```python
from build123d import *

# Parameters (mm, degrees)
BOSS_EXTRUDE1_DEPTH = 10
SKETCH3_R           = 1.75
CUT_EXTRUDE1_DEPTH  = 12.874342087
FILLET2_R           = 1


with BuildPart() as part:
    # Sketch1 → Boss-Extrude1 (new body)
    with BuildSketch(Plane.XY):
        Polygon((-2.5, 0), (2.5, 0), (5, 3), (5, 4), (-5, 4), (-5, 3), align=None)
    extrude(amount=BOSS_EXTRUDE1_DEPTH)

    # Sketch3 → Cut-Extrude1 (cut, through all)
    with BuildSketch(Plane(origin=(0, 4, 0), x_dir=(1, 0, 0), z_dir=(0, 1, 0))):
        with Locations(Location((0, -5, 0), (0, 0, 270))):
            Circle(SKETCH3_R)
    extrude(amount=-CUT_EXTRUDE1_DEPTH, mode=Mode.SUBTRACT)

    # Fillet2
    # the kernel refuses this fillet: 1 mm, written as the material it takes off along each edge
    with BuildSketch(Plane(origin=(-5, 0, 10), x_dir=(0, 0, -1), z_dir=(1, 0, 0))) as fillet2_piece_1:
        with BuildLine():
            CenterArc((FILLET2_R, FILLET2_R), FILLET2_R, 180, 90)
            Line((0, FILLET2_R), (0, 0))
            Line((0, 0), (FILLET2_R, 0))
        make_face()
    extrude(amount=10, mode=Mode.SUBTRACT)
    with BuildSketch(Plane(origin=(0.899539001, -1.920553199, 10), x_dir=(-0.768221279597376, 0.6401843996644797, 0), z_dir=(0.6401843996644797, 0.768221279597376, 0))) as fillet2_piece_2:
        with BuildLine():
            CenterArc((FILLET2_R, -FILLET2_R), FILLET2_R, 90, 90)
            Line((0, -FILLET2_R), (0, 0))
            Line((0, 0), (FILLET2_R, 0))
        make_face()
    extrude(amount=8.905124838, mode=Mode.SUBTRACT)
    with BuildSketch(Plane(origin=(-6.600460999, 4.920553199, 10), x_dir=(0, 0, -1), z_dir=(0.6401843996644797, -0.768221279597376, 0))) as fillet2_piece_3:
        with BuildLine():
            CenterArc((FILLET2_R, FILLET2_R), FILLET2_R, 180, 90)
            Line((0, FILLET2_R), (0, 0))
            Line((0, 0), (FILLET2_R, 0))
        make_face()
    extrude(amount=8.905124838, mode=Mode.SUBTRACT)
    with BuildSketch(Plane(origin=(7.5, 4, 10), x_dir=(0, -1, 0), z_dir=(-1, 0, 0))) as fillet2_piece_4:
        with BuildLine():
            CenterArc((FILLET2_R, -FILLET2_R), FILLET2_R, 90, 90)
            Line((0, -FILLET2_R), (0, 0))
            Line((0, 0), (FILLET2_R, 0))
        make_face()
    extrude(amount=15, mode=Mode.SUBTRACT)
    with BuildSketch(Plane(origin=(0, 4, 5), x_dir=(0, 0, 1), z_dir=(-1, 0, 0))) as fillet2_piece_5:
        with BuildLine():
            CenterArc((1.75 + FILLET2_R, -FILLET2_R), FILLET2_R, 90, 90)
            Line((1.75 + FILLET2_R, 0), (1.75, 0))
            Line((1.75, 0), (1.75, -FILLET2_R))
        make_face()
    revolve(axis=Axis((0, 4, 5), (0, 1, 0)), mode=Mode.SUBTRACT)


solid = part.part
```
Model file for the job. Use its own axes, mm. Give positions to 0.01 mm unless a question says otherwise; leave off trailing zeros. Write each loop counter-clockwise with the first axis right and the second up, starting at its lowest first coordinate (ties: lowest second). Pieces come first, ordered by that corner, then holes. Notation, with made-up numbers: (18, 80.25) - (33, 80.25) arc R21 ccw to (33, 89.25) - close; hole circle Ø11 at (25, -7.5). An arc over 180 degrees is marked (long way). One line per question, with ' | ' between items. Start each with the question number.
(1) Two-plate mould, pull along X, no slides. Class faces 1 (the face through (0.07, 3.699, 9.715)), 2 (the face through (0.08, 1.52, 3.25)), 3 (the face through (-3.689, 1.896, 9.715)), 4 (the face through (3.732, 1.479, 4.437)): +X half, -X half, draft (parallel to the pull), parting line (faces both ways), or undercut.
(2) Slice it at B-B on x = 0. Write the cut outline in (y, z), plus the area to 3 significant figures.
(3) Wall check: line 1 along X through (y, z) = (2.1, 5); line 2 along X through (y, z) = (2.1, 6.5); line 3 along Y through (x, z) = (2.75, 6). Give the ranges that are in metal, low to high. Write a range as from..to.
(4) Slice it at A-A on z = 5. Write the cut outline in (x, y), plus the area to 3 significant figures.
(5) Pin check, flat tip, straight feed: P1, Ø3, axis at x = 0, z = 5, coming from the -Y side (3 decimals). Stop position of the tip, or through.
Results below:
1) face 1: draft | face 2: undercut | face 3: -X half | face 4: +X half
2) outline: (0, 0) - (4, 0) - (4, 2.25) arc R1 ccw to (3, 3.25) - (0, 3.25) - close; (0, 6.75) - (3, 6.75) arc R1 ccw to (4, 7.75) - (4, 9) arc R1 ccw to (3, 10) - (1, 10) arc R1 ccw to (0, 9) - close | area: 25.1 mm^2
3) line 1: -4.25..-1.75, 1.75..4.25 | line 2: -4.25..-0.9, 0.9..4.25 | line 3: 0.3..4
4) outline: (-5, 3) - (-2.5, 0) - (-1.75, 0) - (-1.75, 3) arc R1 ccw to (-2.75, 4) - (-5, 4) - close; (1.75, 0) - (2.5, 0) - (5, 3) - (5, 4) - (2.75, 4) arc R1 ccw to (1.75, 3) - close | area: 18.1 mm^2
5) P1: through
